Read the model definition and answer for the solid it produces. Units are mm, in the model's axes. A direction names the side the tool comes from. Round coordinates to 2 decimals unless told otherwise and drop trailing zeros. Loops run counter-clockwise (first coordinate to the right, second up) from the corner with the lowest first, then second, coordinate; pieces in that order, holes last. Notation, with made-up numbers: M -33,-1.75 L -25,-1.75 A18 ccw -25,14.25 Z; hole C -30,88.25 d1. An arc over 180 degrees is marked long. Write each question's results on one line, items separated by ' | '.
```python
from build123d import *

# Parameters (mm, degrees)
SKETCH_1_R          = 19.325
SKETCH_1_R_2        = 2.5
EXTRUDE_1_DEPTH     = 16
SKETCH_2_R          = 22.5
SKETCH_2_R_2        = 2.5
EXTRUDE_2_DEPTH     = 2
SKETCH_3_R          = 22.5
SKETCH_3_R_2        = 2.5
EXTRUDE_3_DEPTH     = 2
CUT_EXTRUDE_1_REACH = 22


with BuildPart() as part:
    # 草图1 → 凸台-拉伸1 (new body)
    with BuildSketch(Plane(origin=(0, 0, 0), x_dir=(1, 0, 0), z_dir=(0, 1, 0))):
        Circle(SKETCH_1_R)
        Circle(SKETCH_1_R_2, mode=Mode.SUBTRACT)
    extrude(amount=EXTRUDE_1_DEPTH)

    # 草图2 → 凸台-拉伸2 (add)
    with BuildSketch(Plane(origin=(0, 16, 0), x_dir=(1, 0, 0), z_dir=(0, 1, 0))):
        Circle(SKETCH_2_R)
        Circle(SKETCH_2_R_2, mode=Mode.SUBTRACT)
    extrude(amount=EXTRUDE_2_DEPTH)

    # 草图3 → 凸台-拉伸3 (add)
    with BuildSketch(Plane.XZ):
        Circle(SKETCH_3_R)
        Circle(SKETCH_3_R_2, mode=Mode.SUBTRACT)
    extrude(amount=EXTRUDE_3_DEPTH)

    # 草图4 → 切除-拉伸1 (cut, up to next)
    with BuildSketch(Plane(origin=(0, 18, 0), x_dir=(1, 0, 0), z_dir=(0, 1, 0)), mode=Mode.PRIVATE) as cut_extrude_1_sk1:
        with BuildLine():
            Line((-3.469870315, 3.6), (3.469870315, 3.6))
            ThreePointArc((3.469870315, 3.6), (0, -5), (-3.469870315, 3.6))
        make_face()
    cut_extrude_1_tool1 = extrude(cut_extrude_1_sk1.sketch, amount=-CUT_EXTRUDE_1_REACH, mode=Mode.PRIVATE) & part.part
    add(cut_extrude_1_tool1.solids().sort_by_distance((0, 18, 0.387599))[0], mode=Mode.SUBTRACT)


solid = part.part
```
1. Which of the six approach directions +Z, -Z, +X, -X, +Y, -Y give full straight-line access (tool end or side, diameter ignored) to faces 1 (the face through (0, 8, -3.6)), 2 (the face through (-19.306, 7.888, -0.85)), 3 (the face through (0, -2, -5))?
Completed:
face 1: +Y, -Y | face 2: none | face 3: +Z, -Z, +X, -X, -Y
2. Determine the mould class of faces 4 (the face through (0, 18, -5)), 5 (the face through (10.382, -0.986, -19.961)), 6 (the face through (0, 8, 5)) for opening direction Z: released by +Z, released by -Z, zero draft, split by the parting line, or undercut.
Completed:
face 4: zero draft | face 5: split by the parting line | face 6: undercut
3. Given P1, Ø4, axis at y = 1.5, z = -15, coming from the +X side; P2, Ø16, axis at x = 0, z = 0, coming from the -Y side; P3, Ø6, axis at y = 11.5, z = -3.5, coming from the +X side; P4, Ø8, axis at y = 0.5, z = 9, coming from the -X side, each flat-ended and moving along its own axis, determine where each tip first touches the part or whether it passes through.
Completed:
P1: stops at x = 17.87 | P2: stops at y = -2 | P3: stops at x = 19.32 | P4: stops at x = -21.93
4. Find section C-C, the plane y = 10.5. Give the vertices of the cut face in (x, z) (3 decimals).
Completed:
outline: C 0,0 d38.65; hole M -3.47,-3.6 L 3.47,-3.6 A5 ccw long Z
5. Find the intervals of material crossed by L1, parallel to Z at x = 0, y = 11.25 (3 decimals); L2, parallel to X at y = 13, z = 0 (3 decimals); L3, parallel to X at y = 12.75, z = -2, in increasing order.
Completed:
L1: z = -19.325 to -3.6, 5 to 19.325 | L2: x = -19.325 to -5, 5 to 19.325 | L3: x = -19.22 to -4.58, 4.58 to 19.22
6. Find section A-A, the plane z = 0. Give the vertices of the cut face in (x, y) (3 decimals).
Completed:
outline: M -22.5,-2 L -5,-2 L -5,18 L -22.5,18 L -22.5,16 L -19.325,16 L -19.325,0 L -22.5,0 Z; M 5,-2 L 22.5,-2 L 22.5,0 L 19.325,0 L 19.325,16 L 22.5,16 L 22.5,18 L 5,18 Z
7. Find section D-D, the plane x = 9. Give the vertices of the cut face in (y, z).
Completed:
outline: M -2,-20.62 L 0,-20.62 L 0,-17.1 L 16,-17.1 L 16,-20.62 L 18,-20.62 L 18,20.62 L 16,20.62 L 16,17.1 L 0,17.1 L 0,20.62 L -2,20.62 Z
8. Find section B-B, the plane x = 0. Give the vertices of the cut face in (y, z) (3 decimals), then the cut area to 3 significant figures.
Completed:
outline: M -2,-22.5 L 0,-22.5 L 0,-19.325 L 16,-19.325 L 16,-22.5 L 18,-22.5 L 18,-3.6 L -2,-3.6 Z; M -2,5 L 18,5 L 18,22.5 L 16,22.5 L 16,19.325 L 0,19.325 L 0,22.5 L -2,22.5 Z | area: 626 mm2
